The listing builds one solid part. Answer for the finished solid, in the listing's coordinates (mm). Give positions to 0.01 mm unless a question says otherwise; leave off trailing zeros. Write each loop counter-clockwise with the first axis right and the second up, starting at its lowest first coordinate (ties: lowest second). Pieces come first, ordered by that corner, then holes.
```python
from build123d import *

# Parameters (mm, degrees)
CROQUIS1_W              = 190
CROQUIS1_H              = 70
SALIENTE_EXTRUIR1_DEPTH = 3
CROQUIS2_R              = 2
CROQUIS2_W              = 130
CROQUIS2_H              = 20
CORTAR_EXTRUIR1_DEPTH   = 3
REDONDEO1_R             = 7


with BuildPart() as part:
    # Croquis1 → Saliente-Extruir1 (new body)
    with BuildSketch(Plane(origin=(0, 0, 0), x_dir=(1, 0, 0), z_dir=(0, 1, 0))):
        with Locations((95, -35)):
            Rectangle(CROQUIS1_W, CROQUIS1_H)
    extrude(amount=SALIENTE_EXTRUIR1_DEPTH)

    # Croquis2 → Cortar-Extruir1 (cut)
    with BuildSketch(Plane(origin=(0, 3, 0), x_dir=(1, 0, 0), z_dir=(0, 1, 0))):
        with Locations(Location((15, -8, 0), (0, 0, 270))):
            Circle(CROQUIS2_R)
        with Locations(Location((175, -8, 0), (0, 0, 270))):
            Circle(CROQUIS2_R)
        with Locations(Location((175, -62, 0), (0, 0, 270))):
            Circle(CROQUIS2_R)
        with Locations(Location((15, -62, 0), (0, 0, 270))):
            Circle(CROQUIS2_R)
        with Locations((95, -10)):
            Rectangle(CROQUIS2_W, CROQUIS2_H)
        with Locations((95, -60)):
            Rectangle(CROQUIS2_W, CROQUIS2_H)
    extrude(amount=-CORTAR_EXTRUIR1_DEPTH, mode=Mode.SUBTRACT)

    # Redondeo1
    redondeo1_edges = [part.edges().sort_by_distance(p)[0] for p in [
        (30, 1.5, 70),
        (160, 1.5, 70),
        (30, 1.5, 0),
        (160, 1.5, 0),
        (0, 1.5, 0),
        (190, 1.5, 0),
        (190, 1.5, 70),
        (0, 1.5, 70),
    ]]
    fillet(redondeo1_edges, radius=REDONDEO1_R)


solid = part.part
```
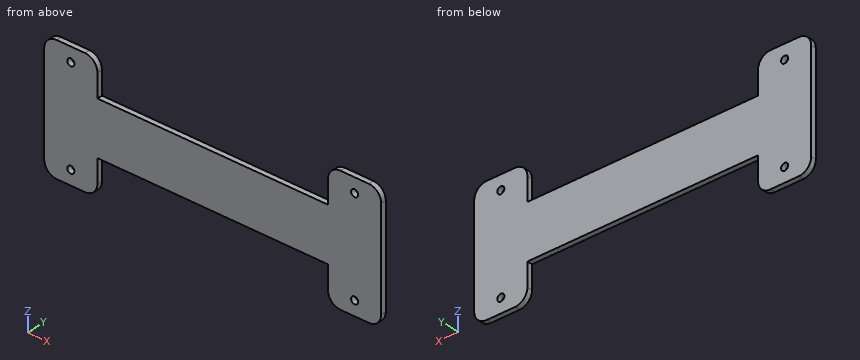
Item 1: A cutting plane is placed at A-A, the plane x = 15. Give the vertices of the cut face in (y, z), plus the area to 3 significant figures.
Conclusion:
outline: (0, 0) - (3, 0) - (3, 6) - (0, 6) - close; (0, 10) - (3, 10) - (3, 60) - (0, 60) - close; (0, 64) - (3, 64) - (3, 70) - (0, 70) - close
area: 186 mm2
Item 2: This flat-tipped pin is pushed along its axis until it touches: P1, Ø4.5, axis at x = 175, z = 8, coming from the -Y side. Where does it stop, or does it pass through?
Conclusion:
P1: stops at y = 0
Item 3: A cutting plane is placed at C-C, the plane x = 87. Give the vertices of the cut face in (y, z), plus the area to 3 significant figures.
Conclusion:
outline: (0, 20) - (3, 20) - (3, 50) - (0, 50) - close
area: 90.0 mm2
Item 4: Consider probe 1 along X at (y, z) = (0.9, 62); probe 2 along Z at (x, y) = (175, 1.75); probe 3 along X at (y, z) = (1.3, 59.5). Determine where each line is inside the solid, lowest interval first.
Conclusion:
probe 1: x = 0 to 13, 17 to 30, 160 to 173, 177 to 190
probe 2: z = 0 to 6, 10 to 60, 64 to 70
probe 3: x = 0 to 30, 160 to 190
Item 5: A cutting plane is placed at B-B, the plane y = 2.1. Give the vertices of the cut face in (x, z).
Conclusion:
outline: (0, 7) arc R7 ccw to (7, 0) - (23, 0) arc R7 ccw to (30, 7) - (30, 20) - (160, 20) - (160, 7) arc R7 ccw to (167, 0) - (183, 0) arc R7 ccw to (190, 7) - (190, 63) arc R7 ccw to (183, 70) - (167, 70) arc R7 ccw to (160, 63) - (160, 50) - (30, 50) - (30, 63) arc R7 ccw to (23, 70) - (7, 70) arc R7 ccw to (0, 63) - close; hole circle Ø4 at (15, 8); hole circle Ø4 at (15, 62); hole circle Ø4 at (175, 8); hole circle Ø4 at (175, 62)
